Geometry check sheet. Reference: the model listing, model coordinates, mm. A direction names the side the tool comes from. Coordinates: 2 decimals unless noted, no trailing zeros. Write each loop counter-clockwise with the first axis right and the second up, starting at its lowest first coordinate (ties: lowest second). Pieces come first, ordered by that corner, then holes. Notation, with made-up numbers: (46, -27) -> (60, -27) arc R16 ccw to (60, 0) -> close; hole circle Ø8 at (4.25, 48.5). An arc over 180 degrees is marked (long way). Answer as CSV lines item,"result".
```python
from build123d import *

# Parameters (mm, degrees)
SKETCH1_W           = 60
SKETCH1_H           = 60
BOSS_EXTRUDE1_DEPTH = 6
CUT_EXTRUDE2_DEPTH  = 3
SKETCH12_R          = 1.15
CUT_EXTRUDE9_DEPTH  = 43.848570571
SKETCH5_W           = 20
SKETCH5_H           = 60
BOSS_EXTRUDE2_DEPTH = 7
SKETCH6_R           = 1.15
CUT_EXTRUDE4_DEPTH  = 45.373415465
CUT_EXTRUDE6_DEPTH  = 10
SKETCH10_W          = 6
SKETCH10_H          = 33.5
CUT_EXTRUDE7_DEPTH  = 3
CUT_EXTRUDE8_DEPTH  = 66.711490624
SKETCH13_W          = 60
SKETCH13_H          = 60
BOSS_EXTRUDE3_DEPTH = 6
SKETCH14_R          = 1.15
CUT_EXTRUDE10_DEPTH = 82.908485519
SKETCH15_R          = 2.2
CUT_EXTRUDE11_DEPTH = 2


with BuildPart() as part:
    # Sketch1 → Boss-Extrude1 (new body)
    with BuildSketch(Plane.XY):
        Rectangle(SKETCH1_W, SKETCH1_H)
    extrude(amount=BOSS_EXTRUDE1_DEPTH)

    # Sketch3 → Cut-Extrude2 (cut)
    with BuildSketch(Plane(origin=(0, 0, 0), x_dir=(-1, 0, 0), z_dir=(0, 0, -1))):
        Polygon((2.1, 6.287564435), (2.1, 8.712435565), (0, 9.924871131), (-2.1, 8.712435565), (-2.1, 6.287564435), (0, 5.075128869), align=None)
        Polygon((2.1, -8.712435565), (2.1, -6.287564435), (0, -5.075128869), (-2.1, -6.287564435), (-2.1, -8.712435565), (0, -9.924871131), align=None)
        Polygon((2.1, -23.712435565), (2.1, -21.287564435), (0, -20.075128869), (-2.1, -21.287564435), (-2.1, -23.712435565), (0, -24.924871131), align=None)
        Polygon((0, 20.075128869), (2.1, 21.287564435), (2.1, 23.712435565), (0, 24.924871131), (-2.1, 23.712435565), (-2.1, 21.287564435), align=None)
    extrude(amount=-CUT_EXTRUDE2_DEPTH, mode=Mode.SUBTRACT)

    # Sketch12 → Cut-Extrude9 (cut, through all)
    with BuildSketch(Plane(origin=(0, 0, 0), x_dir=(-1, 0, 0), z_dir=(0, 0, -1))):
        with Locations((0, 22.5)):
            Circle(SKETCH12_R)
        with Locations((0, 7.5)):
            Circle(SKETCH12_R)
        with Locations((0, -7.5)):
            Circle(SKETCH12_R)
        with Locations((0, -22.5)):
            Circle(SKETCH12_R)
    extrude(amount=-CUT_EXTRUDE9_DEPTH, mode=Mode.SUBTRACT)

    # Sketch5 → Boss-Extrude2 (add)
    with BuildSketch(Plane.XY.offset(6)):
        with Locations((-20, 0)):
            Rectangle(SKETCH5_W, SKETCH5_H)
        with Locations((20, 0)):
            Rectangle(SKETCH5_W, SKETCH5_H)
    extrude(amount=BOSS_EXTRUDE2_DEPTH)

    # Sketch6 → Cut-Extrude4 (cut, through all)
    with BuildSketch(Plane.XY.offset(13)):
        with Locations((-25, 25)):
            Circle(SKETCH6_R)
        with Locations((25, 25)):
            Circle(SKETCH6_R)
        with Locations((25, -25)):
            Circle(SKETCH6_R)
        with Locations((-25, -25)):
            Circle(SKETCH6_R)
    extrude(amount=-CUT_EXTRUDE4_DEPTH, mode=Mode.SUBTRACT)

    # Sketch9 → Cut-Extrude6 (cut)
    with BuildSketch(Plane.XY.offset(13)):
        Polygon((-25, -16.55), (-15.5, -27), (-10, -27), (-10, 6.5), (-23.375, 6.5), (-25, 4.9), (-25, 3.3), (-27, 3.3), (-27, -3.3), (-25, -3.3), align=None)
    extrude(amount=-CUT_EXTRUDE6_DEPTH, mode=Mode.SUBTRACT)

    # Sketch10 → Cut-Extrude7 (cut)
    with BuildSketch(Plane.XY.offset(6)):
        with Locations((-7, -10.25)):
            Rectangle(SKETCH10_W, SKETCH10_H)
    extrude(amount=-CUT_EXTRUDE7_DEPTH, mode=Mode.SUBTRACT)

    # Sketch11 → Cut-Extrude8 (cut, through all)
    with BuildSketch(Plane(origin=(-27, 0, 0), x_dir=(0, 0, -1), z_dir=(1, 0, 0))):
        with BuildLine():
            Line((-3, -0.899652711), (-3, 0.899652711))
            ThreePointArc((-3, 0.899652711), (-9.475, 0), (-3, -0.899652711))
        make_face()
    extrude(amount=-CUT_EXTRUDE8_DEPTH, mode=Mode.SUBTRACT)

    # Sketch13 → Boss-Extrude3 (add)
    with BuildSketch(Plane(origin=(0, -30, 0), x_dir=(-1, 0, 0), z_dir=(0, -1, 0))):
        with Locations((0, -17)):
            Rectangle(SKETCH13_W, SKETCH13_H)
    extrude(amount=BOSS_EXTRUDE3_DEPTH)

    # Sketch14 → Cut-Extrude10 (cut, through all)
    with BuildSketch(Plane(origin=(0, -30, 0), x_dir=(1, 0, 0), z_dir=(0, 1, 0))):
        with BuildLine():
            ThreePointArc((-25.813172798, 8.813172798), (-25.813172798, 7.186827202), (-24.186827202, 7.186827202))
            Line((-24.186827202, 7.186827202), (-25.813172798, 8.813172798))
        make_face()
        with BuildLine():
            Line((-25.813172798, 8.813172798), (-24.186827202, 7.186827202))
            ThreePointArc((-24.186827202, 7.186827202), (-23.937538538, 7.559914053), (-23.85, 8))
            ThreePointArc((-23.85, 8), (-24.559914053, 9.062461462), (-25.813172798, 8.813172798))
        make_face()
        with Locations(Location((25, 8, 0), (0, 0, 270))):
            Circle(SKETCH14_R)
        with BuildLine():
            ThreePointArc((26.15, -42), (25.440085947, -40.937538538), (24.186827202, -41.186827202))
            Line((24.186827202, -41.186827202), (25.813172798, -42.813172798))
            ThreePointArc((25.813172798, -42.813172798), (26.062461462, -42.440085947), (26.15, -42))
        make_face()
        with BuildLine():
            Line((25.813172798, -42.813172798), (24.186827202, -41.186827202))
            ThreePointArc((24.186827202, -41.186827202), (24.186827202, -42.813172798), (25.813172798, -42.813172798))
        make_face()
        with Locations(Location((-25, -42, 0), (0, 0, 270))):
            Circle(SKETCH14_R)
    extrude(amount=-CUT_EXTRUDE10_DEPTH, mode=Mode.SUBTRACT)

    # Sketch15 → Cut-Extrude11 (cut)
    with BuildSketch(Plane(origin=(0, -30, 0), x_dir=(1, 0, 0), z_dir=(0, 1, 0))):
        with Locations(Location((25, -42, 0), (0, 0, 270))):
            Circle(SKETCH15_R)
        with Locations(Location((-25, -42, 0), (0, 0, 270))):
            Circle(SKETCH15_R)
        with Locations(Location((-25, 8, 0), (0, 0, 270))):
            Circle(SKETCH15_R)
        with Locations(Location((25, 8, 0), (0, 0, 270))):
            Circle(SKETCH15_R)
    extrude(amount=-CUT_EXTRUDE11_DEPTH, mode=Mode.SUBTRACT)


solid = part.part
```
Item 1: Cross-section at D-D, the plane z = 27. Record the cut outline in (x, y).
Responses:
outline,"(-30, -36) -> (30, -36) -> (30, -30) -> (-30, -30) -> close"
Item 2: Cross-section at C-C, the plane y = 7.5. Record the cut outline in (x, z), plus the area to 4 significant figures.
Responses:
outline,"(-30, 0) -> (-2.1, 0) -> (-2.1, 3) -> (-1.15, 3) -> (-1.15, 6) -> (-10, 6) -> (-10, 13) -> (-30, 13) -> close; (1.15, 3) -> (2.1, 3) -> (2.1, 0) -> (30, 0) -> (30, 13) -> (10, 13) -> (10, 6) -> (1.15, 6) -> close"
area,"620.5 mm2"
Item 3: Cross-section at B-B, the plane x = 21. Record the cut outline in (y, z), plus the area to 3 significant figures.
Responses:
outline,"(-36, -13) -> (-30, -13) -> (-30, 0) -> (30, 0) -> (30, 13) -> (-30, 13) -> (-30, 47) -> (-36, 47) -> close"
area,"1,140 mm2"
Item 4: Thickness scan on probe 1 along X at (y, z) = (-35.1, 42); probe 2 along Y at (x, z) = (0, 4); probe 3 along X at (y, z) = (-30.65, 42). Record the ranges inside material, lowest first.
Responses:
probe 1,"x = -30 to -26.15, -23.85 to 23.85, 26.15 to 30"
probe 2,"y = -36 to -23.65, -21.35 to -8.65, -6.35 to 6.35, 8.65 to 21.35, 23.65 to 30"
probe 3,"x = -30 to -27.2, -22.8 to 22.8, 27.2 to 30"
Item 5: Cross-section at A-A, the plane y = -7.5. Record the cut outline in (x, z).
Responses:
outline,"(-30, 0) -> (-2.1, 0) -> (-2.1, 3) -> (-1.15, 3) -> (-1.15, 6) -> (-4, 6) -> (-4, 3) -> (-25, 3) -> (-25, 13) -> (-30, 13) -> close; (1.15, 3) -> (2.1, 3) -> (2.1, 0) -> (30, 0) -> (30, 13) -> (10, 13) -> (10, 6) -> (1.15, 6) -> close"
Item 6: Set-up check for faces 1 (the flat face through (-26, 3.3, 8)), 2 (the flat face through (2.1, -22, 1)), 3 (the flat face through (-26, -32, -7)): record each of +Z, -Z, +X, -X, +Y, -Y from which the full face is reachable in a straight line by a thin tool's end or side.
Responses:
face 1,"+Z"
face 2,"-Z"
face 3,"+Y"
Item 7: Depth check by flat-ended pin: pin 1 Ø2.5 at (x, z) = (-25, -8) entering from +Y; pin 2 Ø22 at (x, y) = (-22, 7.5) entering from +Z; pin 3 Ø1.3 at (x, y) = (-0.5, 8) entering from -Z. Enter the tip coordinate at first touch or a pass-through.
Responses:
pin 1,"stops at y = -32"
pin 2,"stops at z = 13"
pin 3,"stops at z = 3"
Item 8: Release check for a two-part mould opening along Z. For faces 4 (the flat face through (0, -9, 3)), 5 (the cylindrical face through (23.98, -33.97, -7.47)), 6 (the cylindrical face through (0.15, -6.36, 4.48)) record: +Z half, -Z half, draft (parallel to the pull), parting line (faces both ways), or undercut.
Responses:
face 4,"-Z half"
face 5,"undercut"
face 6,"draft"
